For this review, use the dimensioned drawing (mm, ordinates from the lowest corner) and the shaded views. A direction names the side the tool comes from. Round coordinates to 2 decimals unless told otherwise and drop trailing zeros. Write each loop counter-clockwise with the first axis right and the second up, starting at its lowest first coordinate (ties: lowest second). Pieces come first, ordered by that corner, then holes. Notation, with made-up numbers: (-34.75, 77.25) - (-16.75, 77.25) arc R25 cw to (-16.75, 100.25) - close; hole circle Ø1 at (52.25, 53.25). An arc over 180 degrees is marked (long way). Write each question's results on one line, items separated by ' | '.
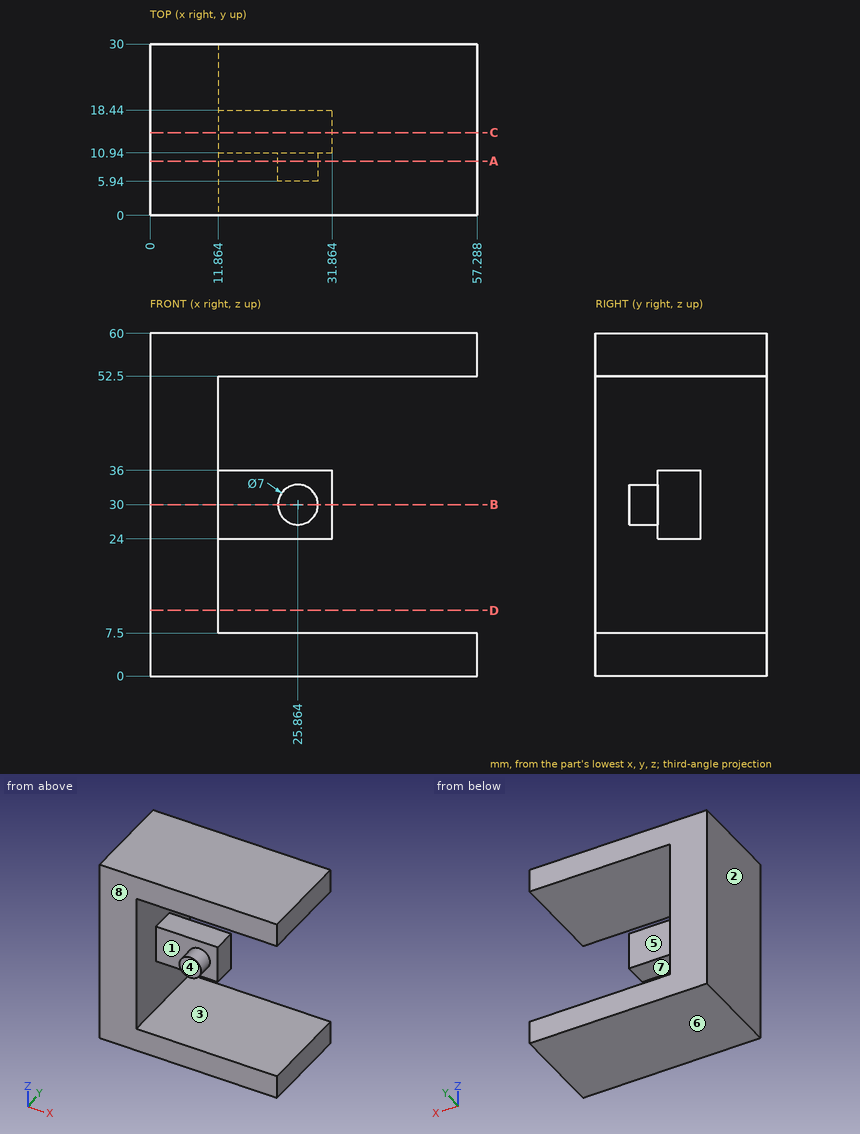
Q1. Tool access review of the marked faces 4, 5, 6, 7 and 8: name each direction out of +Z, -Z, +X, -X, +Y, -Y from which nothing blocks a thin tool from reaching the whole face with its end or side.
Evaluation:
face 4: +X, -Y | face 5: +X, +Y | face 6: -Z, +X, -X, +Y, -Y | face 7: +X, +Y, -Y | face 8: +Z, -Z, +X, -X, -Y
Q2. We need section B-B (z = 30). State the section outline as (x, y) points (1 decimal), plus the area to 3 significant figures.
Evaluation:
outline: (0, 0) - (11.9, 0) - (11.9, 10.9) - (22.4, 10.9) - (22.4, 5.9) - (29.4, 5.9) - (29.4, 10.9) - (31.9, 10.9) - (31.9, 18.4) - (11.9, 18.4) - (11.9, 30) - (0, 30) - close | area: 541 mm^2
Q3. Insertion check: P1, Ø1.5, axis at x = 13, z = 27.5, coming from the +Y side; P2, Ø2, axis at y = 16, z = 31, coming from the +X side; P3, Ø3.5, axis at x = 25, z = 29.5, coming from the -Y side. Each pin has a flat end and moves straight along its axis. Give the tip position at first contact, or say it passes through.
Evaluation:
P1: stops at y = 18.44 | P2: stops at x = 31.86 | P3: stops at y = 5.94
Q4. For probe 1 along Z at (x, y) = (14, 16); probe 2 along Z at (x, y) = (42.5, 6); probe 3 along X at (y, z) = (1.75, 12.5) (1 decimal), list the stretches that pass through material, from the lowest coordinate up.
Evaluation:
probe 1: z = 0 to 7.5, 24 to 36, 52.5 to 60 | probe 2: z = 0 to 7.5, 52.5 to 60 | probe 3: x = 0 to 11.9
Q5. We need section D-D (z = 11.5). State the section outline as (x, y) points (1 decimal).
Evaluation:
outline: (0, 0) - (11.9, 0) - (11.9, 30) - (0, 30) - close
Q6. We need section A-A (y = 9.5). State the section outline as (x, z) points (1 decimal).
Evaluation:
outline: (0, 0) - (57.3, 0) - (57.3, 7.5) - (11.9, 7.5) - (11.9, 52.5) - (57.3, 52.5) - (57.3, 60) - (0, 60) - close; circle Ø7 at (25.9, 30)
Q7. We need section C-C (y = 14.5). State the section outline as (x, z) points (1 decimal), plus the area to 3 significant figures.
Evaluation:
outline: (0, 0) - (57.3, 0) - (57.3, 7.5) - (11.9, 7.5) - (11.9, 24) - (31.9, 24) - (31.9, 36) - (11.9, 36) - (11.9, 52.5) - (57.3, 52.5) - (57.3, 60) - (0, 60) - close | area: 1,630 mm^2
Q8. The part is to be moulded in two halves that separate along X. For the marked faces 1, 2 and 3, say which applies: released by +X, released by -X, zero draft, split by the parting line, or undercut.
Evaluation:
face 1: undercut | face 2: released by -X | face 3: zero draft
